The listing builds one solid part. Answer for the finished solid, in the listing's coordinates (mm). A direction names the side the tool comes from. Give positions to 0.01 mm unless a question says otherwise; leave off trailing zeros. Write each loop counter-clockwise with the first axis right and the second up, starting at its lowest first coordinate (ties: lowest second). Pieces come first, ordered by that corner, then holes. Notation, with made-up numbers: (-16.75, 83.5) - (-7.75, 83.5) arc R26 ccw to (-7.75, 102.5) - close; hole circle Ø4 at (9.5, -23.5). An arc over 180 degrees is marked (long way). Return JSON: item names as keys, results as strings.
Autodesk Inventor part; units mm, degrees
ref_plane "Work Plane1" through (0, 0, 50.8) normal (0, 0, 1) x (1, 0, 0)
ref_plane "YZ Plane" through (0, 0, 0) normal (1, 0, 0) x (0, 1, 0)
ref_plane "XZ Plane" through (0, 0, 0) normal (0, 1, 0) x (-1, 0, 0)
sketch "Sketch2" plane through (0, 0, 0) normal (0, 0, 1) x (1, 0, 0)
  line L0 (0, 0) -> (25.4, 0)
  line L1 (25.4, 0) -> (25.4, 5.588)
  line L2 (25.4, 5.588) -> (0, 5.588)
  line L3 (0, 5.588) -> (0, 0)
  arc A0 (25.4, 0) -> (25.4, 5.588) centre (25.4, 2.794) ccw
  dimension "d0" = 25.4
  dimension "d1" = 5.588
ref_plane "Work Plane1" through (0, 0, 50.8) normal (0, 0, 1) x (1, 0, 0)
sketch "Sketch3" plane through (0, 0, 50.8) normal (0, 0, 1) x (1, 0, 0)
  line L0 (0, 1.2065) -> (6.35, 1.2065)
  line L1 (6.35, 1.2065) -> (6.35, 4.3815)
  line L2 (6.35, 4.3815) -> (0, 4.3815)
  line L3 (0, 4.3815) -> (0, 1.2065)
  arc A0 (6.35, 1.2065) -> (6.35, 4.3815) centre (6.35, 2.794) ccw
  point P0 (0, 0)
  dimension "d3" = 6.35
  dimension "d4" = 3.175
  dimension "d5" = 1.2065
loft "Loft1" add profiles "Sketch2", "Sketch3"
sketch "Sketch4" plane through (0, 0, 0) normal (-1, 0, 0) x (0, 0, 1)
  line L0 (0, 5.588) -> (0, 0)
  line L1 (0, 0) -> (50.8, 1.2065)
  line L2 (50.8, 4.3815) -> (50.8, 1.2065)
  line L3 (0, 5.588) -> (50.8, 4.3815)
  line L4 (0, 5.588) -> (50.8, 4.3815)
  line L5 (44.45, 4.5323) -> (44.45, 1.0557)
  line L6 (50.8, 1.2065) -> (0, 0)
  dimension "d10" = 6.35
extrude "Extrusion1" add sketch "Sketch4" along normal blind 38.608 contours L3 L2 L1 L5
sketch "Sketch5" plane through (25.4, 5.588, 0) normal (0, 0, -1) x (-1, 0, 0)
  line L0 (25.4, 0) -> (25.4, -5.588)
  line L1 (0, 0) -> (25.4, 0)
  arc A0 (0, 0) -> (0, -5.588) centre (0, -2.794) ccw
  line L2 (25.4, -5.588) -> (0, -5.588)
  line L3 (25.4, 0) -> (25.4, -5.588)
  line L4 (25.4, 0) -> (36.1487, 0)
  line L5 (36.1487, 0) -> (36.1487, -5.5776)
  line L6 (36.1487, -5.5776) -> (25.4, -5.5776)
  line L7 (25.4, -5.5776) -> (25.4, 0)
  line L8 (-3.175, -0.1076) -> (-3.175, -7.007)
  line L9 (25.4, -5.588) -> (0, -5.588)
revolve "Revolution1" add sketch "Sketch5" angle 15 about axis through (28.575, 5.4804, 0) along (0, -1, 0)
sketch "Sketch7" plane through (-10.7487, 5.588, 0) normal (0, 1, 0) x (1, 0, 0)
  line L0 (0, 0) -> (10.7487, 0)
  line L1 (36.1487, 0) -> (10.7487, 0)
  arc A0 (36.2569, 0.8218) -> (36.1487, 0) centre (39.3237, 0) ccw
  line L2 (1.3399, 10.1777) -> (36.2569, 0.8218)
  arc A1 (1.3399, 10.1777) -> (0, 0) centre (39.3237, 0) ccw
  line L3 (10.7487, 0) -> (10.7487, -44.45)
  line L4 (10.7487, 0) -> (-2.0556, 0)
  line L5 (-2.0556, 0) -> (-2.0556, 10.6947)
  line L6 (-2.0556, 10.6947) -> (10.7487, 10.6947)
  line L7 (10.7487, 10.6947) -> (10.7487, 0)
extrude "Extrusion2" cut sketch "Sketch7" against normal blind 38.1 contours A1 L2 L7 L0 | L4 L5 L6 L7 L2 A1
sketch "Sketch8" plane through (0, 0.0104, -7.6566) normal (0.258819, 0, -0.9659258) x (-0.9659258, 0, -0.258819)
  line L0 (-29.583, 2.7836) -> (-24.8205, 2.7836)
  line L1 (-24.8205, 2.7836) -> (-8.9455, 2.7836)
  circle A0 centre (-24.8205, 2.7836) radius 1.27
  circle A1 centre (-8.9455, 2.7836) radius 1.27
  line L2 (-26.408, -0.0104) -> (0, -0.0104)
  point P0 (-1.9817, -0.0104)
  point P1 (0, 0)
  dimension "d17" = 4.7625
  dimension "d18" = 15.875
  dimension "d19" = 2.54
  dimension "d20" = 2.54
  dimension "d23" = 2.794
extrude "Extrusion4" cut sketch "Sketch8" against normal blind 12.7
fillet "Fillet2" radius 1.27 1 edges at (0, 2.794, 44.45)
properties part number "DivePlanesStabilizingFins"
Item 1: Flat-ended cylindrical pins translate along their axes: P1, Ø3, axis at x = -26, y = 2, coming from the -Z side; P2, Ø0.8, axis at x = 0.5, z = -4.5, coming from the -Y side; P3, Ø12, axis at x = 0.5, z = 13, coming from the +Y side; P4, Ø3, axis at y = 2, z = 5.5, coming from the -X side. Find the tip coordinate at first contact, or state that the pin passes through.
Answer below:
{"P1": "stops at z = 44.45", "P2": "stops at y = 0", "P3": "stops at y = 5.42", "P4": "stops at x = 0"}
Item 2: Consider L1, parallel to X at y = 3.3, z = 2.5; L2, parallel to Z at x = -26.5, y = 1.7; L3, parallel to X at y = 3.45, z = 3. Determine where each line is inside the solid, lowest interval first.
Answer below:
{"L1": "x = 0 to 5.33, 7.75 to 21.77, 24.18 to 27.15", "L2": "z = 44.45 to 50.8", "L3": "x = 0 to 5.28, 7.53 to 21.71, 23.97 to 26.92"}
Item 3: A cutting plane is placed at A-A on x = -4. Determine the outline of the cut face in (y, z), then the cut area to 3 significant figures.
Answer below:
{"outline": "(1.06, 44.45) - (4.53, 44.45) - (4.38, 50.8) - (1.21, 50.8) - close", "area": "21.1 mm²"}
Item 4: For faces 4 (the face through (14.301, 2.833, -3.825)), 5 (the face through (20.7, 2.81, 11.04)), 6 (the face through (0, 3, 18)), determine the directions among +Z, -Z, +X, -X, +Y, -Y from which every point of the face is accessible in a straight line to the end or side of a thin tool.
Answer below:
{"face 4": "-Z, +X, +Y, -Y", "face 5": "none", "face 6": "-Z, -X, +Y, -Y"}
Item 5: The mould has two halves that part along X. Classify faces 1 (the face through (5.37, 2.812, 6.932)), 2 (the face through (-15, 3, 50.8)), 3 (the face through (-38.608, 3, 48)): +X half, -X half, draft (parallel to the pull), parting line (faces both ways), or undercut.
Answer below:
{"face 1": "undercut", "face 2": "draft", "face 3": "-X half"}
